from build123d import *

# Parameters (mm, degrees)
SKETCH053_R          = 19.8
SKETCH053_R_2        = 17.75
PAD020_DEPTH         = 15
SKETCH054_W          = 40
SKETCH054_H          = 22
POCKET033_DEPTH      = 15.001
POCKET033_DEPTH_BACK = 15.001
FILLET009_R          = 1


with BuildPart() as part:
    # Sketch053 → Pad020 (new body, symmetric)
    with BuildSketch(Plane.XY):
        Circle(SKETCH053_R)
        Circle(SKETCH053_R_2, mode=Mode.SUBTRACT)
    extrude(amount=PAD020_DEPTH, both=True)

    # Sketch054 → Pocket033 (cut, two sides)
    with BuildSketch(Plane.XY) as pocket033_sk:
        with Locations((0, -9.2)):
            Rectangle(SKETCH054_W, SKETCH054_H)
    extrude(amount=-POCKET033_DEPTH, mode=Mode.SUBTRACT)
    extrude(pocket033_sk.sketch, amount=POCKET033_DEPTH_BACK, mode=Mode.SUBTRACT)

    # Fillet009
    fillet009_edges = [part.edges().sort_by_distance(p)[0] for p in [
        (-19.718012, 1.8, 0),
        (19.718012, 1.8, 0),
    ]]
    fillet(fillet009_edges, radius=FILLET009_R)


solid = part.part
Geometry: final body of the model. Coordinates: model frame, mm. Give positions to 0.01 mm unless a question says otherwise; leave off trailing zeros. Write each loop counter-clockwise with the first axis right and the second up, starting at its lowest first coordinate (ties: lowest second). Pieces come first, ordered by that corner, then holes. Notation, with made-up numbers: M 31,52.25 L 45,52.25 A22 ccw 45,81.25 Z; hole C 35,75.25 d9. An arc over 180 degrees is marked long. Answer in a Markdown table with one row per item. Add a question column.
(1) Section B-B on z = -2. Return loops of the section in (x, y).
(2) First-contact query: pin 1 (1.5 mm diameter, centred on x = -15.5, z = -5.5, fed in from -Y); pin 2 (6 mm diameter, centred on x = 10, y = 13, fed in from +Z); pin 3 (6 mm diameter, centred on x = -0.5, z = -2, fed in from +Y); pin 4 (2 mm diameter, centred on x = 9.5, z = -10.5, fed in from +Y). Flat tips, straight axial feed; report the tip coordinate or a pass-through.
(3) Mould query, pull axis X, two halves, no side actions, for faces 1 (the cylindrical face through (-19.36, 2.16, 0.21)), 2 (the flat face through (-3, 18, -15)), 3 (the cylindrical face through (0.365, 17.746, -0.21)). Classes: +X half, -X half, draft (parallel to the pull), parting line (faces both ways), or undercut.
(4) Section C-C on y = 5.75. Return loops of the section in (x, z).
(5) Section A-A on y = 17.25. Return loops of the section in (x, z).
(6) Section D-D on x = -4. Return loops of the section in (y, z).
(7) Ray query, line 1 (X direction, y = 14.25, z = -2); line 2 (X direction, y = 13.25, z = 3.5); line 3 (Y direction, x = -6.5, z = -9.5). Return the intervals inside material, ascending.
Result set:
| question | item | result |
|---|---|---|
| 1 | outline | M -19.58,2.95 A1 ccw -18.59,1.8 L -17.66,1.8 A17.75 cw 17.66,1.8 L 18.59,1.8 A1 ccw 19.58,2.95 A19.8 ccw Z |
| 2 | pin 1 | stops at y = 7.14 |
| 2 | pin 2 | stops at z = 15 |
| 2 | pin 3 | stops at y = 19.8 |
| 2 | pin 4 | stops at y = 17.88 |
| 3 | face 1 | -X half |
| 3 | face 2 | draft |
| 3 | face 3 | undercut |
| 4 | outline | M -18.95,-15 L -16.79,-15 L -16.79,15 L -18.95,15 Z; M 16.79,-15 L 18.95,-15 L 18.95,15 L 16.79,15 Z |
| 5 | outline | M -9.72,-15 L -4.18,-15 L -4.18,15 L -9.72,15 Z; M 4.18,-15 L 9.72,-15 L 9.72,15 L 4.18,15 Z |
| 6 | outline | M 17.29,-15 L 19.39,-15 L 19.39,15 L 17.29,15 Z |
| 7 | line 1 | x = -13.75 to -10.58, 10.58 to 13.75 |
| 7 | line 2 | x = -14.71 to -11.81, 11.81 to 14.71 |
| 7 | line 3 | y = 16.52 to 18.7 |
